```python
from build123d import *

# Parameters (mm, degrees)
SKETCH_1_W                      = 700
SKETCH_1_H                      = 700
CONNECTION_PLATE_DEPTH          = 8
SKETCH_2_W                      = 76
SKETCH_2_H                      = 300
ACCESS_WINDOW_DEPTH             = 990.981818015
SKETCH_3_W                      = 76
SKETCH_3_H                      = 300
CUT_EXTRUDE_2_DEPTH             = 990.981818015
SKETCH_4_W                      = 76
SKETCH_4_H                      = 300
CUT_EXTRUDE_3_DEPTH             = 990.981818015
SKETCH_5_W                      = 76
SKETCH_5_H                      = 300
CUT_EXTRUDE_4_DEPTH             = 990.981818015
SKETCH_6_R                      = 11
SHAFT_CLEARANCE_DEPTH           = 990.981818015
SKETCH_7_R                      = 11
CUT_EXTRUDE_6_DEPTH             = 990.981818015
SKETCH_8_R                      = 11
CUT_EXTRUDE_7_DEPTH             = 990.981818015
SKETCH_9_R                      = 11
CUT_EXTRUDE_8_DEPTH             = 990.981818015
SKETCH_10_R                     = 11
CUT_EXTRUDE_9_DEPTH             = 990.981818015
SKETCH_11_R                     = 11
CUT_EXTRUDE_10_DEPTH            = 990.981818015
SKETCH_12_R                     = 11
CUT_EXTRUDE_11_DEPTH            = 990.981818015
SKETCH_13_R                     = 11
CUT_EXTRUDE_12_DEPTH            = 990.981818015
SKETCH_14_R                     = 11
CUT_EXTRUDE_13_DEPTH            = 990.981818015
SKETCH_15_R                     = 11
CUT_EXTRUDE_14_DEPTH            = 990.981818015
SKETCH_16_R                     = 11
CUT_EXTRUDE_15_DEPTH            = 990.981818015
SKETCH_17_R                     = 11
CUT_EXTRUDE_16_DEPTH            = 990.981818015
SKETCH_18_W                     = 384
SKETCH_18_H                     = 604
FLOAT_INSTALLATION_WINDOW_DEPTH = 990.981818015


with BuildPart() as part:
    # 草图1 → Connection_plate (new body)
    with BuildSketch(Plane.XY):
        with Locations((350, 350)):
            Rectangle(SKETCH_1_W, SKETCH_1_H)
    extrude(amount=CONNECTION_PLATE_DEPTH)

    # 草图2 → Access_window (cut, through all)
    with BuildSketch(Plane.XY.offset(8)):
        with Locations((273, 175)):
            Rectangle(SKETCH_2_W, SKETCH_2_H)
    extrude(amount=-ACCESS_WINDOW_DEPTH, mode=Mode.SUBTRACT)

    # 草图3 → 切除-拉伸2 (cut, through all)
    with BuildSketch(Plane.XY.offset(8)):
        with Locations((273, 525)):
            Rectangle(SKETCH_3_W, SKETCH_3_H)
    extrude(amount=-CUT_EXTRUDE_2_DEPTH, mode=Mode.SUBTRACT)

    # 草图4 → 切除-拉伸3 (cut, through all)
    with BuildSketch(Plane.XY.offset(8)):
        with Locations((427, 175)):
            Rectangle(SKETCH_4_W, SKETCH_4_H)
    extrude(amount=-CUT_EXTRUDE_3_DEPTH, mode=Mode.SUBTRACT)

    # 草图5 → 切除-拉伸4 (cut, through all)
    with BuildSketch(Plane.XY.offset(8)):
        with Locations((427, 525)):
            Rectangle(SKETCH_5_W, SKETCH_5_H)
    extrude(amount=-CUT_EXTRUDE_4_DEPTH, mode=Mode.SUBTRACT)

    # 草图6 → Shaft_clearance (cut, through all)
    with BuildSketch(Plane.XY.offset(8)):
        with Locations((48, 51)):
            Circle(SKETCH_6_R)
    extrude(amount=-SHAFT_CLEARANCE_DEPTH, mode=Mode.SUBTRACT)

    # 草图7 → 切除-拉伸6 (cut, through all)
    with BuildSketch(Plane.XY.offset(8)):
        with Locations((48, 243)):
            Circle(SKETCH_7_R)
    extrude(amount=-CUT_EXTRUDE_6_DEPTH, mode=Mode.SUBTRACT)

    # 草图8 → 切除-拉伸7 (cut, through all)
    with BuildSketch(Plane.XY.offset(8)):
        with Locations((48, 457)):
            Circle(SKETCH_8_R)
    extrude(amount=-CUT_EXTRUDE_7_DEPTH, mode=Mode.SUBTRACT)

    # 草图9 → 切除-拉伸8 (cut, through all)
    with BuildSketch(Plane.XY.offset(8)):
        with Locations((48, 649)):
            Circle(SKETCH_9_R)
    extrude(amount=-CUT_EXTRUDE_8_DEPTH, mode=Mode.SUBTRACT)

    # 草图10 → 切除-拉伸9 (cut, through all)
    with BuildSketch(Plane.XY.offset(8)):
        with Locations((103.43, 147)):
            Circle(SKETCH_10_R)
    extrude(amount=-CUT_EXTRUDE_9_DEPTH, mode=Mode.SUBTRACT)

    # 草图11 → 切除-拉伸10 (cut, through all)
    with BuildSketch(Plane.XY.offset(8)):
        with Locations((103.43, 553)):
            Circle(SKETCH_11_R)
    extrude(amount=-CUT_EXTRUDE_10_DEPTH, mode=Mode.SUBTRACT)

    # 草图12 → 切除-拉伸11 (cut, through all)
    with BuildSketch(Plane.XY.offset(8)):
        with Locations((652, 51)):
            Circle(SKETCH_12_R)
    extrude(amount=-CUT_EXTRUDE_11_DEPTH, mode=Mode.SUBTRACT)

    # 草图13 → 切除-拉伸12 (cut, through all)
    with BuildSketch(Plane.XY.offset(8)):
        with Locations((652, 243)):
            Circle(SKETCH_13_R)
    extrude(amount=-CUT_EXTRUDE_12_DEPTH, mode=Mode.SUBTRACT)

    # 草图14 → 切除-拉伸13 (cut, through all)
    with BuildSketch(Plane.XY.offset(8)):
        with Locations((652, 457)):
            Circle(SKETCH_14_R)
    extrude(amount=-CUT_EXTRUDE_13_DEPTH, mode=Mode.SUBTRACT)

    # 草图15 → 切除-拉伸14 (cut, through all)
    with BuildSketch(Plane.XY.offset(8)):
        with Locations((652, 649)):
            Circle(SKETCH_15_R)
    extrude(amount=-CUT_EXTRUDE_14_DEPTH, mode=Mode.SUBTRACT)

    # 草图16 → 切除-拉伸15 (cut, through all)
    with BuildSketch(Plane.XY.offset(8)):
        with Locations((596.57, 147)):
            Circle(SKETCH_16_R)
    extrude(amount=-CUT_EXTRUDE_15_DEPTH, mode=Mode.SUBTRACT)

    # 草图17 → 切除-拉伸16 (cut, through all)
    with BuildSketch(Plane.XY.offset(8)):
        with Locations((596.57, 553)):
            Circle(SKETCH_17_R)
    extrude(amount=-CUT_EXTRUDE_16_DEPTH, mode=Mode.SUBTRACT)

    # 草图18 → Float_installation_window (cut, through all)
    with BuildSketch(Plane.XY.offset(8)):
        with Locations((350, 350)):
            Rectangle(SKETCH_18_W, SKETCH_18_H)
    extrude(amount=-FLOAT_INSTALLATION_WINDOW_DEPTH, mode=Mode.SUBTRACT)


solid = part.part
```
Build history of the part. All positions in model axes, mm. Round coordinates to 2 decimals unless told otherwise and drop trailing zeros. Order: outer loops, then holes, each group sorted by start corner. A loop starts at its lowest first (then second) coordinate and runs counter-clockwise, first axis right, second up. Notation, with made-up numbers: (69, -5) -> (108, -5) arc R5 ccw to (108, 4) -> close; hole circle Ø1 at (-18.75, 69). An arc over 180 degrees is marked (long way). Answer in a Markdown table with one row per item.
1) Band-saw the part on B-B on y = 243. Give the cut face in (x, z), and give its area (3 significant figures).
Values:
| item | result |
|---|---|
| outline | (0, 0) -> (37, 0) -> (37, 8) -> (0, 8) -> close; (59, 0) -> (158, 0) -> (158, 8) -> (59, 8) -> close; (542, 0) -> (641, 0) -> (641, 8) -> (542, 8) -> close; (663, 0) -> (700, 0) -> (700, 8) -> (663, 8) -> close |
| area | 2,180 mm2 |
2) Wall check: L1, parallel to X at y = 649, z = 5; L2, parallel to Y at x = 103.43, z = 4.5; L3, parallel to X at y = 553, z = 3. Give the ranges that are in metal, low to high.
Values:
| item | result |
|---|---|
| L1 | 0 to 37, 59 to 158, 542 to 641, 663 to 700 |
| L2 | 0 to 136, 158 to 542, 564 to 700 |
| L3 | 0 to 92.43, 114.43 to 158, 542 to 585.57, 607.57 to 700 |
3) Mould opens along X. For faces 1 (the flat face through (112, 355, 8)), 2 (the cylindrical face through (662.161, 452.787, 4.056)) say: released by +X, released by -X, zero draft, split by the parting line, or undercut.
Values:
| item | result |
|---|---|
| face 1 | zero draft |
| face 2 | undercut |
4) Band-saw the part on A-A on x = 652. Give the cut face in (y, z), and give its area (3 significant figures).
Values:
| item | result |
|---|---|
| outline | (0, 0) -> (40, 0) -> (40, 8) -> (0, 8) -> close; (62, 0) -> (232, 0) -> (232, 8) -> (62, 8) -> close; (254, 0) -> (446, 0) -> (446, 8) -> (254, 8) -> close; (468, 0) -> (638, 0) -> (638, 8) -> (468, 8) -> close; (660, 0) -> (700, 0) -> (700, 8) -> (660, 8) -> close |
| area | 4,900 mm2 |
5) Band-saw the part on C-C on x = 103.43. Give the cut face in (y, z).
Values:
| item | result |
|---|---|
| outline | (0, 0) -> (136, 0) -> (136, 8) -> (0, 8) -> close; (158, 0) -> (542, 0) -> (542, 8) -> (158, 8) -> close; (564, 0) -> (700, 0) -> (700, 8) -> (564, 8) -> close |
